Design review of the part built by this model. Coordinates are the model's own, in mm. Round coordinates to 2 decimals unless told otherwise and drop trailing zeros. Loops run counter-clockwise (first coordinate to the right, second up) from the corner with the lowest first, then second, coordinate; pieces in that order, holes last. Notation, with made-up numbers: (2, -31.75) - (48, -31.75) arc R19 cw to (48, -8.75) - close; hole circle Ø7 at (62.25, 35.25). An arc over 180 degrees is marked (long way). Return JSON: item names as keys, results as strings. Group by question number.
(1) We need section A-A, the plane z = 132.5. Write out the cut boundary in (x, y), and give its area (3 significant figures).
(2) Clearance check with a flat-ended pin moving along its axis: pin 1 (3 mm diameter, centred on x = 336, z = 139.5, fed in from -Y). State where the tip first meets the part, or that it passes through.
(3) We need section B-B, the plane y = 140.5. Write out the cut boundary in (x, z).
(4) Wall thickness on L1, parallel to Z at x = 36, y = 227.5: over which ranges is the line inside the solid? List them lowest first. Write a range as [from, to].
(5) We need section C-C, the plane x = 41.5. Write out the cut boundary in (y, z), and give its area (3 significant figures).
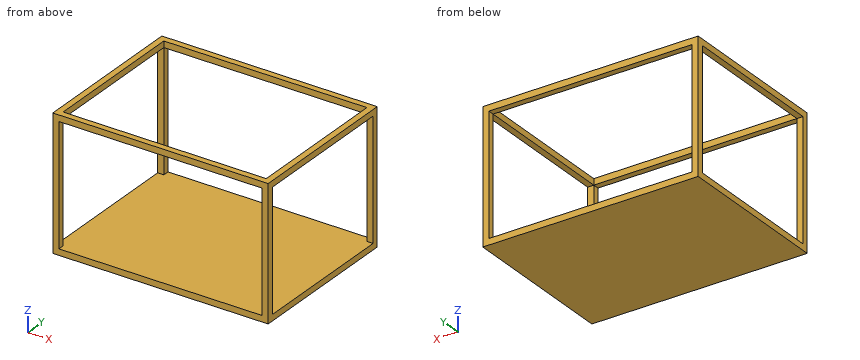
from build123d import *

# Parameters (mm, degrees)
F0_W      = 350
F0_H      = 215
F0_W_2    = 330
F0_H_2    = 195
F2_DEPTH  = 10
F1_W      = 260
F1_H      = 215
F1_W_2    = 240
F1_H_2    = 195
F3_DEPTH  = 10
F4_W      = 340
F4_H      = 240
F5_DEPTH  = 10
F8_W      = 350
F8_H      = 215
F8_W_2    = 330
F8_H_2    = 195
F10_DEPTH = 10
F9_W      = 260
F9_H      = 215
F9_W_2    = 240
F9_H_2    = 195
F11_DEPTH = 10


# Not quite as in the source:
# - a pattern or mirror of a feature is missing from the dataset's text; its kind, count and spacing are read off the source's solid


with BuildPart() as f2:
    # F0 (on Front) → F2 (new body, through all)
    with BuildSketch(Plane.XZ):
        with Locations((165, 97.5)):
            Rectangle(F0_W, F0_H)
        with Locations((165, 97.5)):
            Rectangle(F0_W_2, F0_H_2, mode=Mode.SUBTRACT)
    extrude(amount=-F2_DEPTH)


with BuildPart() as f2_copies_1:
    # F2_copies: instance of F2
    add(f2.part.mirror(Plane.ZX.offset(130)))


with BuildPart() as f2_1:
    add(f2.part)

    add(f2_copies_1.part)  # F3 merges F2_copies_1
    # F1 (on Right) → F3 (join, through all)
    with BuildSketch(Plane.YZ):
        with Locations((130, 97.5)):
            Rectangle(F1_W, F1_H)
        with Locations((130, 97.5)):
            Rectangle(F1_W_2, F1_H_2, mode=Mode.SUBTRACT)
    extrude(amount=-F3_DEPTH)

    # F4 (on face) → F5 (join, through all)
    with BuildSketch(Plane(origin=(0, 0, -10), x_dir=(1, 0, 0), z_dir=(0, 0, -1))):
        Polygon((340, -10), (340, 0), (-10.0000000001, 0), (-10.0000000001, -260), (340, -260), (340, -250), (0, -250), (0, -10), align=None)
        with Locations((170, -130)):
            Rectangle(F4_W, F4_H)
    extrude(amount=-F5_DEPTH)

    # F8 (on plane+point) → F10 (join, through all)
    with BuildSketch(Plane.XZ.offset(-260)):
        with Locations((165, 97.5)):
            Rectangle(F8_W, F8_H)
        with Locations((165, 97.5)):
            Rectangle(F8_W_2, F8_H_2, mode=Mode.SUBTRACT)
    extrude(amount=F10_DEPTH)

    # F9 (on plane+point) → F11 (join, through all)
    with BuildSketch(Plane.YZ.offset(340)):
        with Locations((130, 97.5)):
            Rectangle(F9_W, F9_H)
        with Locations((130, 97.5)):
            Rectangle(F9_W_2, F9_H_2, mode=Mode.SUBTRACT)
    extrude(amount=-F11_DEPTH)


solid = f2_1.part
Solutions:
{
 "1": {"outline": "(-10, 0) - (0, 0) - (0, 10) - (-10, 10) - close; (-10, 250) - (0, 250) - (0, 260) - (-10, 260) - close; (330, 0) - (340, 0) - (340, 10) - (330, 10) - close; (330, 250) - (340, 250) - (340, 260) - (330, 260) - close", "area": "400 mm^2"},
 "2": {"pin 1": "y = 0"},
 "3": {"outline": "(-10, -10) - (340, -10) - (340, 0) - (-10, 0) - close; (-10, 195) - (0, 195) - (0, 205) - (-10, 205) - close; (330, 195) - (340, 195) - (340, 205) - (330, 205) - close"},
 "4": {"L1": "[-10, 0]"},
 "5": {"outline": "(0, -10) - (260, -10) - (260, 0) - (0, 0) - close; (0, 195) - (10, 195) - (10, 205) - (0, 205) - close; (250, 195) - (260, 195) - (260, 205) - (250, 205) - close", "area": "2,800 mm^2"}
}
